Verification items for the finished model (mm, model axes). Face numbers are marked on the shaded views. A direction names the side the tool comes from. Coordinates: 2 decimals unless noted, no trailing zeros. Order: outer loops, then holes, each group sorted by start corner. A loop starts at its lowest first (then second) coordinate and runs counter-clockwise, first axis right, second up.
Q1. Depth check by flat-ended pin: P1, Ø10, axis at y = 27, z = 32.5, coming from the -X side (3 decimals); P2, Ø2, axis at y = 15.5, z = 47, coming from the +X side (3 decimals); P3, Ø2, axis at x = 20, y = 17, coming from the +Z side; P4, Ø2.5, axis at x = 53.975, z = 66.675, coming from the -Y side. Enter the tip coordinate at first touch or a pass-through.
Q2. Cross-section at C-C, the plane y = 16. Record the boundary of the cut face in (x, z) (3 decimals).
Q3. Cross-section at B-B, the plane x = 15. Record the boundary of the cut face in (y, z), and give its area (3 significant figures).
Q4. Set-up check for the marked faces 1, 2 and 3: record each of +Z, -Z, +X, -X, +Y, -Y from which the full face is reachable in a straight line by a thin tool's end or side.
Q5. Cross-section at D-D, the plane x = 51. Record the boundary of the cut face in (y, z).
Q6. Cross-section at A-A, the plane z = 34.5. Record the boundary of the cut face in (x, y) (3 decimals).
Q7. Thickness scan on line 1 (X direction, y = 12, z = 66); line 2 (Z direction, x = -21, y = 25); line 3 (Y direction, x = 56, z = 43). Record the ranges inside material, lowest first.
from build123d import *

# Parameters (mm, degrees)
SKETCH1_W                    = 127
SKETCH1_H                    = 12.7
BOSS_EXTRUDE1_DEPTH          = 76.2
BOSS_EXTRUDE3_DEPTH          = 50.8
F_1_8_0_125_DIAMETER_HOLE1_D = 3.175


with BuildPart() as part:
    # Sketch1 → Boss-Extrude1 (new body)
    with BuildSketch(Plane.XY):
        with Locations((0, 6.35)):
            Rectangle(SKETCH1_W, SKETCH1_H)
    extrude(amount=BOSS_EXTRUDE1_DEPTH)

    # Sketch2 → Boss-Extrude3 (add)
    with BuildSketch(Plane(origin=(0, 0, 0), x_dir=(-1, 0, 0), z_dir=(0, 0, -1))):
        Polygon((-41.275, 12.7), (41.275, 12.7), (41.275, 25.4), (19.277954744, 38.1), (-19.277954744, 38.1), (-41.275, 25.4), align=None)
    extrude(amount=-BOSS_EXTRUDE3_DEPTH)

    # 1/8 (0.125) Diameter Hole1 (through all)
    with Locations(Plane(origin=(0, 12.7, 0), x_dir=(1, 0, 0), z_dir=(0, 1, 0))):
        with Locations((53.975, -9.525), (-53.975, -9.525), (-53.975, -66.675), (53.975, -66.675)):
            Hole(F_1_8_0_125_DIAMETER_HOLE1_D / 2)


solid = part.part
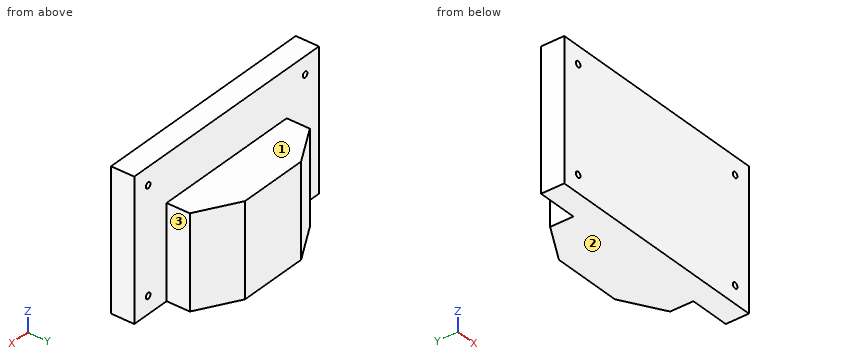
Check values:
1. P1: stops at x = -41.275
1. P2: stops at x = 41.275
1. P3: stops at z = 50.8
1. P4: passes through
2. outline: (-41.275, 0) - (41.275, 0) - (41.275, 50.8) - (-41.275, 50.8) - close
3. outline: (0, 0) - (38.1, 0) - (38.1, 50.8) - (12.7, 50.8) - (12.7, 76.2) - (0, 76.2) - close
3. area: 2,260 mm2
4. face 1: +Z, +X, -X, +Y
4. face 2: -Z, +X, -X, +Y, -Y
4. face 3: +Z, -Z, +X, +Y
5. outline: (0, 0) - (12.7, 0) - (12.7, 76.2) - (0, 76.2) - close
6. outline: (-63.5, 0) - (63.5, 0) - (63.5, 12.7) - (41.275, 12.7) - (41.275, 25.4) - (19.278, 38.1) - (-19.278, 38.1) - (-41.275, 25.4) - (-41.275, 12.7) - (-63.5, 12.7) - close
7. line 1: x = -63.5 to -55.41, -52.54 to 52.54, 55.41 to 63.5
7. line 2: z = 0 to 50.8
7. line 3: y = 0 to 12.7
